Part model, mm, in its own coordinate system. A direction names the side the tool comes from. Give positions to 0.01 mm unless a question says otherwise; leave off trailing zeros. Write each loop counter-clockwise with the first axis right and the second up, starting at its lowest first coordinate (ties: lowest second). Pieces come first, ordered by that corner, then holes. Notation, with made-up numbers: M 54.25,-8.75 L 104.25,-8.75 A19 ccw 104.25,23.25 Z; hole C 63.5,73 d6. An arc over 180 degrees is marked long. Use a Markdown table: item, result.
```python
from build123d import *

# Parameters (mm, degrees)
BOSS_EXTRUDE1_DEPTH     = 10
SKETCH2_R               = 5
CUT_EXTRUDE4_DEPTH      = 11
CUT_EXTRUDE4_DEPTH_BACK = 1
SKETCH3_R               = 7
CUT_EXTRUDE5_DEPTH      = 11


with BuildPart() as part:
    # Sketch1 → Boss-Extrude1 (new body)
    with BuildSketch(Plane(origin=(0, 0, 0), x_dir=(1, 0, 0), z_dir=(0, 1, 0))):
        with BuildLine():
            Line((5, 0), (87.1, 0))
            ThreePointArc((87.1, 0), (94.171067812, 2.928932188), (97.1, 10))
            Line((97.1, 10), (97.1, 63.297208828))
            ThreePointArc((97.1, 63.297208828), (96.949532816, 65.025416948), (96.502659338, 66.701617347))
            ThreePointArc((96.502659338, 66.701617347), (62.853663281, 110.72240479), (10.046495568, 127.5))
            Line((10.046495568, 127.5), (-34.953504432, 127.079547292))
            ThreePointArc((-34.953504432, 127.079547292), (-38.861917641, 126.217874558), (-42.119413536, 123.892601626))
            Line((-42.119413536, 123.892601626), (-132.321113421, 26.947294417))
            ThreePointArc((-132.321113421, 26.947294417), (-134.306211211, 23.795285131), (-135, 20.135444575))
            Line((-135, 20.135444575), (-135, -30))
            ThreePointArc((-135, -30), (-132.071067812, -37.071067812), (-125, -40))
            Line((-125, -40), (-15, -40))
            ThreePointArc((-15, -40), (-7.928932188, -37.071067812), (-5, -30))
            Line((-5, -30), (-5, -10))
            ThreePointArc((-5, -10), (-2.071067812, -2.928932188), (5, 0))
        make_face()
    extrude(amount=BOSS_EXTRUDE1_DEPTH)

    # Sketch2 → Cut-Extrude4 (cut, two sides)
    with BuildSketch(Plane(origin=(0, 0, 0), x_dir=(1, 0, 0), z_dir=(0, 1, 0))) as cut_extrude4_sk:
        with Locations((14.998992834, 111.984631039)):
            Circle(SKETCH2_R)
        with Locations((82.1, 65)):
            Circle(SKETCH2_R)
        with Locations((32.1, 65)):
            Circle(SKETCH2_R)
    extrude(amount=CUT_EXTRUDE4_DEPTH, mode=Mode.SUBTRACT)
    extrude(cut_extrude4_sk.sketch, amount=-CUT_EXTRUDE4_DEPTH_BACK, mode=Mode.SUBTRACT)

    # Sketch3 → Cut-Extrude5 (cut, through all)
    with BuildSketch(Plane.XZ):
        with Locations((-69.615384615, 30)):
            Circle(SKETCH3_R)
    extrude(amount=-CUT_EXTRUDE5_DEPTH, mode=Mode.SUBTRACT)


solid = part.part
```
1. Drill centre lines: L1, parallel to X at y = 3.75, z = 17.5; L2, parallel to Z at x = 32.1, y = 3.5; L3, parallel to Z at x = 83.5, y = 8.5. Where is each one in solid material? Low to high.
Findings below:
| item | result |
|---|---|
| L1 | -135 to -5 |
| L2 | -124.77 to -70, -60 to 0 |
| L3 | -90.72 to -69.8, -60.2 to 0 |
2. Cut at D-D, the plane z = -102. Give the cut face in (x, y).
Findings below:
| item | result |
|---|---|
| outline | M -62.49,0 L 73.48,0 L 73.48,10 L -62.49,10 Z |
3. Tool access for faces 1 (the flat face through (-5, 5, 20)), 2 (the cylindrical face through (84.788, 4.93, -69.216)): list every direction of +Z, -Z, +X, -X, +Y, -Y with a clear straight run to the whole face (end or side of a thin tool).
Findings below:
| item | result |
|---|---|
| face 1 | +Z, +X, +Y, -Y |
| face 2 | +Y, -Y |
4. Cut at C-C, the plane z = -30.5. Give the cut face in (x, y), then the cut area to 3 significant figures.
Findings below:
| item | result |
|---|---|
| outline | M -129.02,0 L 97.1,0 L 97.1,10 L -129.02,10 Z |
| area | 2,260 mm2 |
5. Drop flat-ended pins along their axis: P1, Ø5, axis at y = 5.5, z = 24.5, coming from the +X side; P2, Ø22.5, axis at x = -69.62, z = 30, coming from the -Y side; P3, Ø2, axis at y = 2, z = -66, coming from the -X side; P4, Ø8, axis at x = 32.1, z = -65, coming from the +Y side. Give the stop position or say it passes through.
Findings below:
| item | result |
|---|---|
| P1 | x = -5 |
| P2 | y = 0 |
| P3 | x = -96.92 |
| P4 | through |
6. Cut at A-A, the plane x = 82.1. Give the cut face in (y, z).
Findings below:
| item | result |
|---|---|
| outline | M 0,-92.54 L 10,-92.54 L 10,-70 L 0,-70 Z; M 0,-60 L 10,-60 L 10,0 L 0,0 Z |
7. Cut at B-B, the plane y = 8. Give the cut face in (x, z).
Findings below:
| item | result |
|---|---|
| outline | M -135,-20.14 A10 ccw -132.32,-26.95 L -42.12,-123.89 A10 ccw -34.95,-127.08 L 10.05,-127.5 A92.18 ccw 96.5,-66.7 A10 ccw 97.1,-63.3 L 97.1,-10 A10 ccw 87.1,0 L 5,0 A10 cw -5,10 L -5,30 A10 ccw -15,40 L -125,40 A10 ccw -135,30 Z; hole C -69.62,30 d14; hole C 15,-111.98 d10; hole C 32.1,-65 d10; hole C 82.1,-65 d10 |
8. Two-plate mould, pull along X, no slides. Class faces 3 (the flat face through (-86.59, 4.93, -76.1)), 4 (the cylindrical face through (94.09, 4.93, -2.85)), 5 (the cylindrical face through (-76.61, 4.93, 30.31)): released by +X, released by -X, zero draft, split by the parting line, or undercut.
Findings below:
| item | result |
|---|---|
| face 3 | released by -X |
| face 4 | released by +X |
| face 5 | undercut |
